Geometry: see drawing. Coordinates: mm, zero at the bounding-box minimum. Coordinates: 2 decimals unless noted, no trailing zeros. Write each loop counter-clockwise with the first axis right and the second up, starting at its lowest first coordinate (ties: lowest second). Pieces come first, ordered by that corner, then holes. Notation, with made-up numbers: M -6,-17 L 28,-17 A26 ccw 28,6 Z; hole C 20.5,69 d10. An arc over 180 degrees is marked long. Write item = value, one per line. Start each with the question number.
1. Pin query (flat end, axial travel): pin 1 Ø6.5 at (x, y) = (22, 17) entering from -Z (3 decimals); pin 2 Ø3 at (x, y) = (24.384, 19.05) entering from +Z; pin 3 Ø4 at (x, z) = (13, 2.5) entering from +Y (3 decimals). Return the tip coordinate at first contact, or that it passes through.
2. Pull-direction query (Y, two-part tool) for the marked faces 1, 2, 3 and 4; classes: pulls with the +Y half, pulls with the -Y half, needs draft (parallel to the pull), parting line crosses it, or undercut.
3. Section query B-B (y = 19.05). Give the number of separate pieces and of enclosed holes in the cut face.
4. Line query: line 1 along Y through (x, z) = (16, 23.5); line 2 along Z through (x, y) = (21, 17) (1 decimal); line 3 along Y through (x, z) = (10.5, 16) (1 decimal). Output: solid intervals per line, ascending.
5. Section query A-A (x = 5.08). Output: boundary loops of the cut face in (y, z) (1 decimal).
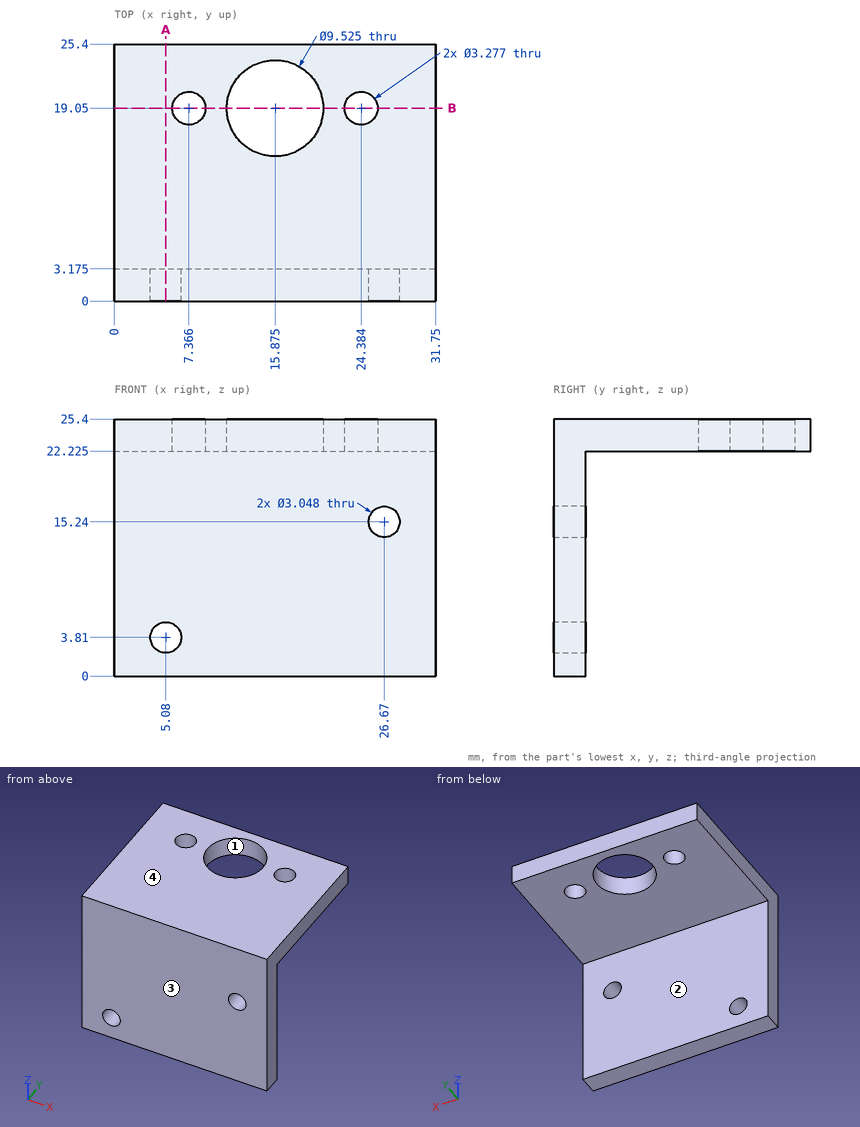
Results are:
q1.pin_1 = 22.225
q1.pin_2 = through
q1.pin_3 = 3.175
q2.face_1 = undercut
q2.face_2 = pulls with the +Y half
q2.face_3 = pulls with the -Y half
q2.face_4 = needs draft
q3.separate_pieces = 4
q3.enclosed_holes = 0
q4.line_1 = 0 to 14.29, 23.81 to 25.4
q4.line_2 = 22.2 to 25.4
q4.line_3 = 0 to 3.2
q5.outline = M 0,0 L 3.2,0 L 3.2,2.3 L 0,2.3 Z; M 0,5.3 L 3.2,5.3 L 3.2,22.2 L 25.4,22.2 L 25.4,25.4 L 0,25.4 Z
